from build123d import *

# Parameters (mm, degrees)
F0_W     = 50.8
F0_H     = 38.1
F1_DEPTH = 31.75
F3_DEPTH = 12.7
F5_DEPTH = 12.7
F7_DEPTH = 25.4


with BuildPart() as f1:
    # F0 (on Top) → F1 (new body)
    with BuildSketch(Plane.XY):
        with Locations((25.4, 19.05)):
            Rectangle(F0_W, F0_H)
    extrude(amount=F1_DEPTH)

    # F2 (on face) → F3 (cut)
    with BuildSketch(Plane.XZ):
        Polygon((19.05, 31.75), (31.75, 0), (50.8, 0), (50.8, 31.75), align=None)
    extrude(amount=-F3_DEPTH, mode=Mode.SUBTRACT)

    # F4 (on face) → F5 (cut)
    with BuildSketch(Plane(origin=(0, 38.1, 0), x_dir=(-1, 0, 0), z_dir=(0, 1, 0))):
        Polygon((-50.8, 0), (-31.75, 0), (-19.05, 31.75), (-50.8, 31.75), align=None)
    extrude(amount=-F5_DEPTH, mode=Mode.SUBTRACT)

    # F6 (on face) → F7 (cut)
    with BuildSketch(Plane.XZ.offset(-12.7)):
        Polygon((44.45, 31.75), (50.8, 0), (50.8, 31.75), align=None)
    extrude(amount=-F7_DEPTH, mode=Mode.SUBTRACT)


solid = f1.part
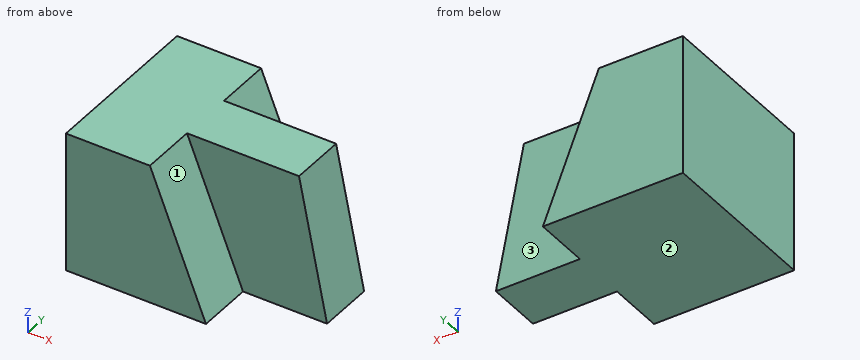
For this review, take the finished solid that the model builds, in its own axes (mm). Face numbers are marked on the shaded views. A direction names the side the tool comes from. Round coordinates to 2 decimals unless told otherwise and drop trailing zeros. Order: outer loops, then holes, each group sorted by start corner. A loop starts at its lowest first (then second) coordinate and runs counter-clockwise, first axis right, second up. Notation, with made-up numbers: M 75,10 L 119,10 A18 ccw 119,23 Z; hole C 20,66.5 d10. An arc over 180 degrees is marked long. Use a Markdown table: item, result. Add a question column.
Item 1: Insertion check: pin 1 (6 mm diameter, centred on x = 38, z = 9.5, fed in from -Y); pin 2 (1 mm diameter, centred on x = 40, z = 28, fed in from +Y); pin 3 (2 mm diameter, centred on y = 7.5, z = 18, fed in from +X). Each pin has a flat end and moves straight along its axis. Give the tip position at first contact, or say it passes through.
Item 2: To check wall thickness, follow line 1 along Y through (x, z) = (26, 16.5); line 2 along X through (y, z) = (3.5, 19); line 3 along X through (y, z) = (31.5, 13.5). State the ranges of each line that lie inside material, in increasing order.
Item 3: Tool access review of the marked faces 1, 2 and 3: name each direction out of +Z, -Z, +X, -X, +Y, -Y from which nothing blocks a thin tool from reaching the whole face with its end or side.
Item 4: Add section C-C, the plane y = 19.5. Give the boundary of the cut face in (x, z).
Item 5: Add section D-D, the plane x = 38. Give the boundary of the cut face in (y, z).
Item 6: Add section B-B, the plane x = 28.5. Give the boundary of the cut face in (y, z) (3 decimals).
Item 7: Add section A-A, the plane z = 15. Give the boundary of the cut face in (x, y).
Geometry results:
| question | item | result |
|---|---|---|
| 1 | pin 1 | stops at y = 12.7 |
| 1 | pin 2 | stops at y = 25.4 |
| 1 | pin 3 | stops at x = 24.95 |
| 2 | line 1 | y = 12.7 to 25.4 |
| 2 | line 2 | x = 0 to 24.15 |
| 2 | line 3 | x = 0 to 26.35 |
| 3 | face 1 | +Z, +X, -Y |
| 3 | face 2 | -Z, +X, -X, +Y, -Y |
| 3 | face 3 | +Z, +X, +Y |
| 4 | outline | M 0,0 L 50.8,0 L 44.45,31.75 L 0,31.75 Z |
| 5 | outline | M 12.7,0 L 25.4,0 L 25.4,31.75 L 12.7,31.75 Z |
| 6 | outline | M 0,0 L 38.1,0 L 38.1,8.125 L 25.4,8.125 L 25.4,31.75 L 12.7,31.75 L 12.7,8.125 L 0,8.125 Z |
| 7 | outline | M 0,0 L 25.75,0 L 25.75,12.7 L 47.8,12.7 L 47.8,25.4 L 25.75,25.4 L 25.75,38.1 L 0,38.1 Z |
